Design review of the part built by this model. Coordinates are the model's own, in mm. Coordinates: 2 decimals unless noted, no trailing zeros. Answer in a Markdown table with one row per item. Add a question column.
(1) We need section A-A, the plane z = 3. Give the number of separate pieces and of enclosed holes in the cut face, plus the area to 3 significant figures.
(2) To check wall thickness, follow L1, parallel to Z at x = 6, y = -0.4; L2, parallel to Z at x = 18, y = -1.3; L3, parallel to Y at x = -4, z = -8. State the ranges of each line that lie inside material, in increasing order. Write a range as [from, to].
(3) Clearance check with flat-ended pins moving along their axes: pin 1 (6.5 mm diameter, centred on x = -12, z = -3, fed in from +Y); pin 2 (4.5 mm diameter, centred on x = 12, z = -3, fed in from -Y). State where each tip first meets the part, or that it passes through.
from build123d import *

# Parameters (mm, degrees)
SKETCH1_W               = 42
SKETCH1_H               = 24
BOSS_EXTRUDE1_DEPTH     = 1.5
FILLET1_R               = 3
SKETCH2_R               = 2
CUT_EXTRUDE1_DEPTH      = 4
SKETCH3_R               = 2.5
CUT_EXTRUDE2_DEPTH      = 0.8
MIRROR2_COPY_1_SKETCH_R = 2.5
MIRROR2_COPY_1_DEPTH    = 0.8


with BuildPart() as part:
    # Sketch1 → Boss-Extrude1 (new body, symmetric)
    with BuildSketch(Plane(origin=(0, 0, 0), x_dir=(1, 0, 0), z_dir=(0, 1, 0))):
        Rectangle(SKETCH1_W, SKETCH1_H)
    extrude(amount=BOSS_EXTRUDE1_DEPTH, both=True)

    # Fillet1
    fillet1_edges = [part.edges().sort_by_distance(p)[0] for p in [
        (-21, 0, -12),
        (21, 0, -12),
        (21, 0, 12),
        (-21, 0, 12),
    ]]
    fillet(fillet1_edges, radius=FILLET1_R)

    # Sketch2 → Cut-Extrude1 (cut, through all)
    with BuildSketch(Plane(origin=(0, 1.5, 0), x_dir=(1, 0, 0), z_dir=(0, 1, 0))):
        with Locations((-18, 9)):
            Circle(SKETCH2_R)
        with Locations((-12, 9)):
            Circle(SKETCH2_R)
        with Locations((-6, 9)):
            Circle(SKETCH2_R)
        with Locations((0, 9)):
            Circle(SKETCH2_R)
        with Locations((6, 9)):
            Circle(SKETCH2_R)
        with Locations((12, 9)):
            Circle(SKETCH2_R)
        with Locations((18, 9)):
            Circle(SKETCH2_R)
        with Locations((-12, 3)):
            Circle(SKETCH2_R)
        with Locations((-6, 3)):
            Circle(SKETCH2_R)
        with Locations((0, 3)):
            Circle(SKETCH2_R)
        with Locations((6, 3)):
            Circle(SKETCH2_R)
        with Locations((12, 3)):
            Circle(SKETCH2_R)
        with Locations((18, 3)):
            Circle(SKETCH2_R)
        with Locations((-12, -3)):
            Circle(SKETCH2_R)
        with Locations((-6, -3)):
            Circle(SKETCH2_R)
        with Locations((0, -3)):
            Circle(SKETCH2_R)
        with Locations((6, -3)):
            Circle(SKETCH2_R)
        with Locations((12, -3)):
            Circle(SKETCH2_R)
        with Locations((18, -3)):
            Circle(SKETCH2_R)
        with Locations((-18, 3)):
            Circle(SKETCH2_R)
        with Locations((-18, -3)):
            Circle(SKETCH2_R)
    cut_extrude1 = extrude(amount=-CUT_EXTRUDE1_DEPTH, mode=Mode.SUBTRACT)

    # Sketch3 → Cut-Extrude2 (cut)
    with BuildSketch(Plane(origin=(0, 1.5, 0), x_dir=(1, 0, 0), z_dir=(0, 1, 0))):
        with Locations((-18, 9)):
            Circle(SKETCH3_R)
        with Locations((-12, 9)):
            Circle(SKETCH3_R)
        with Locations((-6, 9)):
            Circle(SKETCH3_R)
        with Locations((0, 9)):
            Circle(SKETCH3_R)
        with Locations((6, 9)):
            Circle(SKETCH3_R)
        with Locations((12, 9)):
            Circle(SKETCH3_R)
        with Locations((18, 9)):
            Circle(SKETCH3_R)
        with Locations((-12, 3)):
            Circle(SKETCH3_R)
        with Locations((-6, 3)):
            Circle(SKETCH3_R)
        with Locations((0, 3)):
            Circle(SKETCH3_R)
        with Locations((6, 3)):
            Circle(SKETCH3_R)
        with Locations((12, 3)):
            Circle(SKETCH3_R)
        with Locations((18, 3)):
            Circle(SKETCH3_R)
        with Locations((-12, -3)):
            Circle(SKETCH3_R)
        with Locations((-6, -3)):
            Circle(SKETCH3_R)
        with Locations((0, -3)):
            Circle(SKETCH3_R)
        with Locations((6, -3)):
            Circle(SKETCH3_R)
        with Locations((12, -3)):
            Circle(SKETCH3_R)
        with Locations((18, -3)):
            Circle(SKETCH3_R)
        with Locations((-18, 3)):
            Circle(SKETCH3_R)
        with Locations((-18, -3)):
            Circle(SKETCH3_R)
    cut_extrude2 = extrude(amount=-CUT_EXTRUDE2_DEPTH, mode=Mode.SUBTRACT)

    # Mirror1: Cut-Extrude2 across plane
    add(cut_extrude2.mirror(Plane.ZX), mode=Mode.SUBTRACT)

    # Mirror2: Cut-Extrude1, Cut-Extrude2 across plane
    add(cut_extrude1.mirror(Plane.XY), mode=Mode.SUBTRACT)
    add(cut_extrude2.mirror(Plane.XY), mode=Mode.SUBTRACT)

    # Mirror2 copy 1 sketch → Mirror2 copy 1 (cut)
    with BuildSketch(Plane.XZ.offset(1.5)):
        with Locations((-18, 9)):
            Circle(MIRROR2_COPY_1_SKETCH_R)
        with Locations((-12, 9)):
            Circle(MIRROR2_COPY_1_SKETCH_R)
        with Locations((-6, 9)):
            Circle(MIRROR2_COPY_1_SKETCH_R)
        with Locations((0, 9)):
            Circle(MIRROR2_COPY_1_SKETCH_R)
        with Locations((6, 9)):
            Circle(MIRROR2_COPY_1_SKETCH_R)
        with Locations((12, 9)):
            Circle(MIRROR2_COPY_1_SKETCH_R)
        with Locations((18, 9)):
            Circle(MIRROR2_COPY_1_SKETCH_R)
        with Locations((-12, 3)):
            Circle(MIRROR2_COPY_1_SKETCH_R)
        with Locations((-6, 3)):
            Circle(MIRROR2_COPY_1_SKETCH_R)
        with Locations((0, 3)):
            Circle(MIRROR2_COPY_1_SKETCH_R)
        with Locations((6, 3)):
            Circle(MIRROR2_COPY_1_SKETCH_R)
        with Locations((12, 3)):
            Circle(MIRROR2_COPY_1_SKETCH_R)
        with Locations((18, 3)):
            Circle(MIRROR2_COPY_1_SKETCH_R)
        with Locations((-12, -3)):
            Circle(MIRROR2_COPY_1_SKETCH_R)
        with Locations((-6, -3)):
            Circle(MIRROR2_COPY_1_SKETCH_R)
        with Locations((0, -3)):
            Circle(MIRROR2_COPY_1_SKETCH_R)
        with Locations((6, -3)):
            Circle(MIRROR2_COPY_1_SKETCH_R)
        with Locations((12, -3)):
            Circle(MIRROR2_COPY_1_SKETCH_R)
        with Locations((18, -3)):
            Circle(MIRROR2_COPY_1_SKETCH_R)
        with Locations((-18, 3)):
            Circle(MIRROR2_COPY_1_SKETCH_R)
        with Locations((-18, -3)):
            Circle(MIRROR2_COPY_1_SKETCH_R)
    extrude(amount=-MIRROR2_COPY_1_DEPTH, mode=Mode.SUBTRACT)


solid = part.part
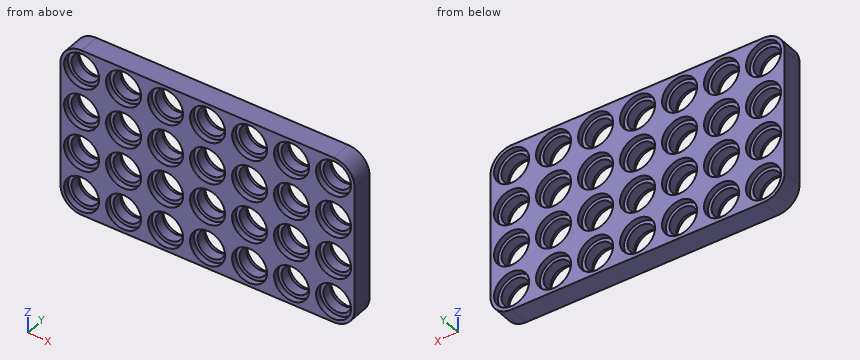
Responses:
| question | item | result |
|---|---|---|
| 1 | separate pieces | 8 |
| 1 | enclosed holes | 0 |
| 1 | area | 30.8 mm2 |
| 2 | L1 | z = [-12, -11], [-7, -5], [-1, 1], [5, 7], [11, 12] |
| 2 | L2 | z = [-12, -11.5], [-6.5, -5.5], [-0.5, 0.5], [5.5, 6.5], [11.5, 12] |
| 2 | L3 | y = [-0.7, 0.7] |
| 3 | pin 1 | stops at y = 1.5 |
| 3 | pin 2 | stops at y = -0.7 |
